```python
from build123d import *

# Parameters (mm, degrees)
F1_W     = 114
F1_H     = 200
F2_DEPTH = 8.65
F3_W     = 94.3653250774
F3_H     = 150.9845201238
F4_DEPTH = 0.1
F5_R     = 5
F6_R     = 4


with BuildPart() as f2:
    # F1 (on Top) → F2 (new body)
    with BuildSketch(Plane.XY):
        Rectangle(F1_W, F1_H)
    extrude(amount=F2_DEPTH)

    # F3 (on face) → F4 (cut)
    with BuildSketch(Plane.XY.offset(8.65)):
        Rectangle(F3_W, F3_H)
    extrude(amount=-F4_DEPTH, mode=Mode.SUBTRACT)

    # F5
    f5_edges = [f2.edges().sort_by_distance(p)[0] for p in [
        (-57, -100, 4.325),
        (57, -100, 4.325),
        (-57, 100, 4.325),
        (57, 100, 4.325),
    ]]
    fillet(f5_edges, radius=F5_R)

    # F6
    f6_edges = [f2.edges().sort_by_distance(p)[0] for p in [
        (-57, 0, 0),
    ]]
    fillet(f6_edges, radius=F6_R)


solid = f2.part
```
Geometry: final body of the model. Coordinates: model frame, mm. Give positions to 0.01 mm unless a question says otherwise; leave off trailing zeros. Loops run counter-clockwise (first coordinate to the right, second up) from the corner with the lowest first, then second, coordinate; pieces in that order, holes last. Notation, with made-up numbers: (11.25, -14.5) -> (26.25, -14.5) arc R22 cw to (26.25, 2.5) -> close; hole circle Ø4 at (36, 41). An arc over 180 degrees is marked (long way). Return JSON: item names as keys, results as strings.
Item 1: Pin query (flat end, axial travel): P1, Ø6, axis at x = -29.5, y = -64.5, coming from the +Z side; P2, Ø1.5, axis at x = 25.5, z = 1.5, coming from the +Y side. Return the tip coordinate at first contact, or that it passes through.
Filled in:
{"P1": "z = 8.55", "P2": "y = 99.6"}
Item 2: Line query: line 1 (Z direction, x = -41.5, y = -53); line 2 (Y direction, x = -50.5, z = 3.5); line 3 (X direction, y = 64, z = 3.5). Output: solid intervals per line, ascending.
Filled in:
{"line 1": "0 to 8.55", "line 2": "-99.97 to 99.97", "line 3": "-56.97 to 56.97"}
Item 3: Section A-A, the plane y = -57. Output: boundary loops of the cut face in (x, z).
Filled in:
{"outline": "(-57, 4) arc R4 ccw to (-53, 0) -> (53, 0) arc R4 ccw to (57, 4) -> (57, 8.65) -> (47.18, 8.65) -> (47.18, 8.55) -> (-47.18, 8.55) -> (-47.18, 8.65) -> (-57, 8.65) -> close"}
